The figure shows three views and two pictorial views of one solid part (mm, origin at its lowest corner). Answer the questions. A direction names the side the tool comes from. Round coordinates to 2 decimals unless told otherwise and drop trailing zeros. Order: outer loops, then holes, each group sorted by start corner. A loop starts at its lowest first (then second) coordinate and runs counter-clockwise, first axis right, second up. Notation, with made-up numbers: (17.25, -25.75) -> (36.25, -25.75) arc R24 ccw to (36.25, 2.25) -> close; hole circle Ø4 at (39.5, 40.25). An arc over 180 degrees is marked (long way). Return JSON: item names as keys, results as strings. Group by question number.
(1) The part is cut by section C-C (y = 15). Determine the outline of the cut face in (x, z), plus the area to 3 significant figures.
(2) The part is cut by section B-B (z = 25). Determine the outline of the cut face in (x, y), plus the area to 3 significant figures.
(3) Which of the six approach directions +Z, -Z, +X, -X, +Y, -Y give full straight-line access (tool end or side, diameter ignored) to the marked faces 1, 2, 3, 4 and 5?
(4) The part is cut by section A-A (x = 16). Determine the outline of the cut face in (y, z).
(5) The part is cut by section D-D (x = 7.7). Determine the outline of the cut face in (y, z).
(6) Consider line 1 (Y direction, x = 7.7, z = 22.55); line 2 (X direction, y = 25.5, z = 15); line 3 (Z direction, x = 3, y = 16.5). Determine where each line is inside the solid, lowest interval first. Write a range as [from, to].
(7) Each of these flat-tipped pins is pushed along its axis until it touches: pin 1 (4 mm diameter, centred on x = 8, y = 5.5, fed in from -Z); pin 2 (5 mm diameter, centred on x = 6.5, z = 26, fed in from +Y); pin 3 (1.6 mm diameter, centred on x = 17.5, z = 15.5, fed in from -Y). Where does it stop, or does it pass through?
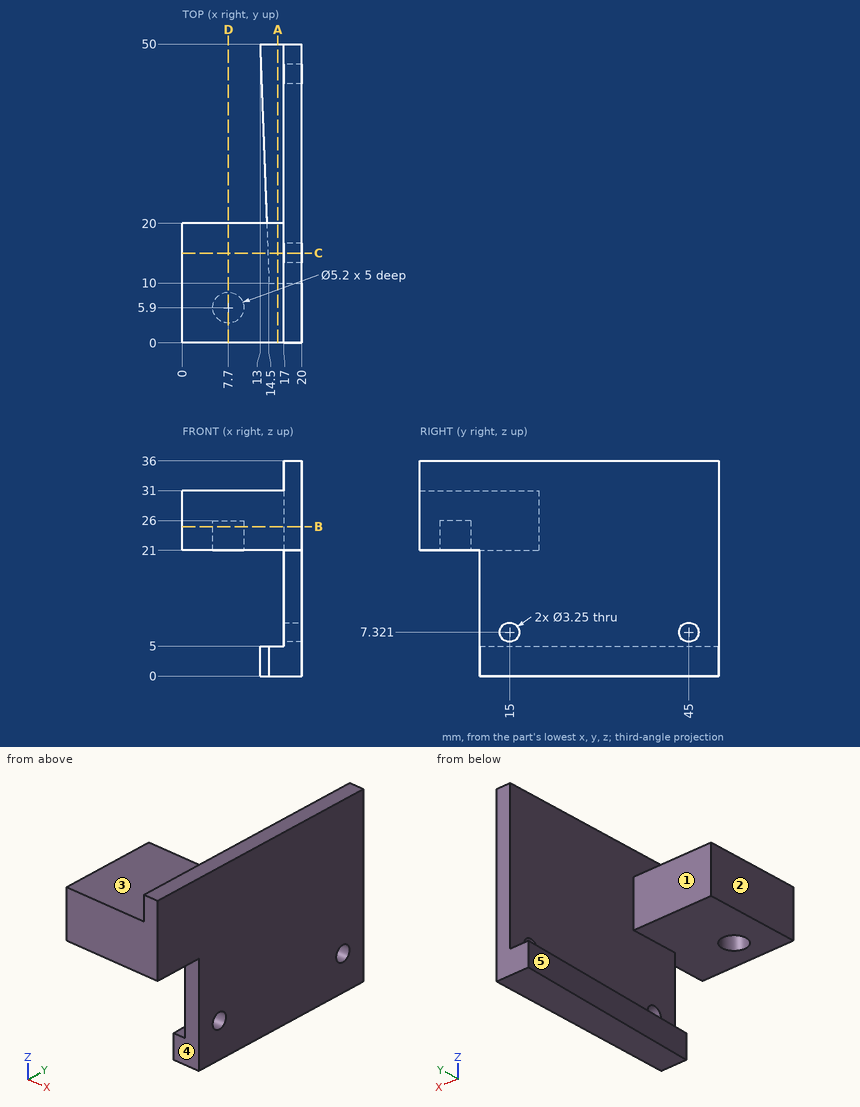
Answer below:
{
 "1": {"outline": "(0, 21) -> (17, 21) -> (17, 8.95) -> (20, 8.95) -> (20, 36) -> (17, 36) -> (17, 31) -> (0, 31) -> close; (14.31, 0) -> (20, 0) -> (20, 5.7) -> (17, 5.7) -> (17, 5) -> (14.31, 5) -> close", "area": "282 mm²"},
 "2": {"outline": "(0, 0) -> (20, 0) -> (20, 50) -> (17, 50) -> (17, 20) -> (0, 20) -> close; hole circle Ø5.2 at (7.7, 5.9)", "area": "469 mm²"},
 "3": {"face 1": "+Z, -X, +Y", "face 2": "+Z, -Z, -X, +Y, -Y", "face 3": "+Z, -X, +Y, -Y", "face 4": "-Z, +X, -X, -Y", "face 5": "-Z, -X, -Y"},
 "4": {"outline": "(0, 21) -> (20, 21) -> (20, 31) -> (0, 31) -> close; (10, 0) -> (50, 0) -> (50, 5) -> (10, 5) -> close"},
 "5": {"outline": "(0, 21) -> (3.3, 21) -> (3.3, 26) -> (8.5, 26) -> (8.5, 21) -> (20, 21) -> (20, 31) -> (0, 31) -> close"},
 "6": {"line 1": "y = [0, 3.3], [8.5, 20]", "line 2": "x = [17, 20]", "line 3": "z = [21, 31]"},
 "7": {"pin 1": "stops at z = 26", "pin 2": "stops at y = 20", "pin 3": "stops at y = 10"}
}
